```python
from build123d import *

# Parameters (mm, degrees)
SKETCH2_W           = 40
SKETCH2_H           = 20
BOSS_EXTRUDE1_DEPTH = 8
CUT_EXTRUDE1_DEPTH  = 9
SKETCH4_R           = 1.7
CUT_EXTRUDE2_DEPTH  = 21
CHAMFER1_SIZE       = 2


with BuildPart() as part:
    # Sketch2 → Boss-Extrude1 (new body)
    with BuildSketch(Plane(origin=(0, 0, 0), x_dir=(1, 0, 0), z_dir=(0, 1, 0))):
        with Locations((20, 10)):
            Rectangle(SKETCH2_W, SKETCH2_H)
    extrude(amount=BOSS_EXTRUDE1_DEPTH)

    # Sketch3 → Cut-Extrude1 (cut, through all)
    with BuildSketch(Plane.XZ):
        with BuildLine():
            Line((12, -8), (12, 0))
            Line((12, 0), (28, 0))
            Line((28, 0), (28, -8))
            ThreePointArc((28, -8), (20, -16), (12, -8))
        make_face()
    extrude(amount=-CUT_EXTRUDE1_DEPTH, mode=Mode.SUBTRACT)

    # Sketch4 → Cut-Extrude2 (cut, through all)
    with BuildSketch(Plane.XY):
        with Locations((7.5, 4)):
            Circle(SKETCH4_R)
        with Locations((32.5, 4)):
            Circle(SKETCH4_R)
    extrude(amount=-CUT_EXTRUDE2_DEPTH, mode=Mode.SUBTRACT)

    # Chamfer1
    chamfer1_edges = [part.edges().sort_by_distance(p)[0] for p in [
        (40, 8, -10),
        (0, 8, -10),
        (40, 0, -10),
        (0, 0, -10),
    ]]
    chamfer(chamfer1_edges, length=CHAMFER1_SIZE)


solid = part.part
```
The model under review builds one solid part; all positions refer to its coordinate system, in mm. A direction names the side the tool comes from. Round coordinates to 2 decimals unless told otherwise and drop trailing zeros. Order: outer loops, then holes, each group sorted by start corner. A loop starts at its lowest first (then second) coordinate and runs counter-clockwise, first axis right, second up.
(1) For P1, Ø1.5, axis at y = 1, z = -15.5, coming from the -X side, flat-tipped, find the tip position at first contact; note if it passes through.
Working result:
P1: stops at x = 0.25
(2) Take a section at B-B, the plane y = 4. State the section outline as (x, z) points, plus the area to 3 significant figures.
Working result:
outline: (0, -20) - (5.8, -20) - (5.8, 0) - (0, 0) - close; (9.2, -20) - (30.8, -20) - (30.8, 0) - (28, 0) - (28, -8) arc R8 cw to (12, -8) - (12, 0) - (9.2, 0) - close; (34.2, -20) - (40, -20) - (40, 0) - (34.2, 0) - close
area: 435 mm2
(3) Tool access review of faces 4 (the face through (35, 4, 0)), 5 (the face through (12, 4, -4)): name each direction out of +Z, -Z, +X, -X, +Y, -Y from which nothing blocks a thin tool from reaching the whole face with its end or side.
Working result:
face 4: +Z, +X, -X, +Y, -Y
face 5: +Z, +Y, -Y
(4) Mouldability with a two-part tool opening along X and no side actions: class faces 1 (the face through (0, 4, -10)), 2 (the face through (39, 1, -10)), 3 (the face through (20, 4, -16)) as released by +X, released by -X, zero draft, split by the parting line, or undercut.
Working result:
face 1: released by -X
face 2: released by +X
face 3: undercut
(5) Take a section at C-C, the plane x = 32.5. State the section outline as (y, z) points, plus the area to 3 significant figures.
Working result:
outline: (0, -20) - (2.3, -20) - (2.3, 0) - (0, 0) - close; (5.7, -20) - (8, -20) - (8, 0) - (5.7, 0) - close
area: 92.0 mm2
(6) Take a section at A-A, the plane z = -6. State the section outline as (x, y) points.
Working result:
outline: (0, 2) - (2, 0) - (12, 0) - (12, 8) - (2, 8) - (0, 6) - close; (28, 0) - (38, 0) - (40, 2) - (40, 6) - (38, 8) - (28, 8) - close; hole circle Ø3.4 at (7.5, 4); hole circle Ø3.4 at (32.5, 4)
(7) Wall thickness on L1, parallel to Y at x = 32.5, z = -11.25; L2, parallel to X at y = 4.75, z = -5.25; L3, parallel to X at y = 2.5, z = -5: over which ranges is each line inside the solid? List them lowest first.
Working result:
L1: y = 0 to 2.3, 5.7 to 8
L2: x = 0 to 5.97, 9.03 to 12, 28 to 30.97, 34.03 to 40
L3: x = 0 to 6.7, 8.3 to 12, 28 to 31.7, 33.3 to 40
(8) Take a section at D-D, the plane y = 7.25. State the section outline as (x, z) points.
Working result:
outline: (1.25, -20) - (38.75, -20) - (38.75, 0) - (28, 0) - (28, -8) arc R8 cw to (12, -8) - (12, 0) - (1.25, 0) - close
